```python
from build123d import *

# Parameters (mm, degrees)
SKETCH1_R                = 1.7526
BOSS_EXTRUDE1_DEPTH      = 6.35
BOSS_EXTRUDE2_DEPTH      = 3.175
BOSS_EXTRUDE2_DEPTH_BACK = 3.175


with BuildPart() as part:
    # Sketch1 → Boss-Extrude1 (new body)
    with BuildSketch(Plane.XY):
        with BuildLine():
            Line((-6.345006919, -1.27), (-6.345006919, 37.592))
            ThreePointArc((-6.345006919, 37.592), (0, 43.937006919), (6.345006919, 37.592))
            Line((6.345006919, 37.592), (6.345006919, -1.27))
            ThreePointArc((6.345006919, -1.27), (0, -7.615006919), (-6.345006919, -1.27))
        make_face()
        Circle(SKETCH1_R, mode=Mode.SUBTRACT)
    extrude(amount=BOSS_EXTRUDE1_DEPTH)

    # Sketch2 → Boss-Extrude2 (add, two sides: drawn at the far end of the back side and taken through both)
    with BuildSketch(Plane(origin=(0, 0, 0), x_dir=(0, 0, -1), z_dir=(1, 0, 0)).offset(-BOSS_EXTRUDE2_DEPTH_BACK)):
        with BuildLine():
            Line((0, 37.592), (0, 24.892))
            Line((0, 24.892), (16.951066371, 27.880930353))
            ThreePointArc((16.951066371, 27.880930353), (18.455752886, 28.749661517), (19.05, 30.382342046))
            Line((19.05, 30.382342046), (19.05, 32.101657954))
            ThreePointArc((19.05, 32.101657954), (18.455752886, 33.734338483), (16.951066371, 34.603069647))
            Line((16.951066371, 34.603069647), (0, 37.592))
        make_face()
    extrude(amount=BOSS_EXTRUDE2_DEPTH + BOSS_EXTRUDE2_DEPTH_BACK)


solid = part.part
```
Design review of the part built by this model. Coordinates are the model's own, in mm. A direction names the side the tool comes from. Give positions to 0.01 mm unless a question says otherwise; leave off trailing zeros. Order: outer loops, then holes, each group sorted by start corner. A loop starts at its lowest first (then second) coordinate and runs counter-clockwise, first axis right, second up. Notation, with made-up numbers: (79, 87.25) -> (104, 87.25) arc R13 cw to (104, 106.25) -> close; hole circle Ø6 at (39, 57.25). An arc over 180 degrees is marked (long way). Write item = value, one per line. Start each with the question number.
(1) We need section B-B on x = 0. Write out the cut boundary in (y, z) (3 decimals), plus the area to 3 significant figures.
(2) We need section A-A on y = 0. Write out the cut boundary in (x, z) (3 decimals).
(3) For faces 1 (the face through (-0.044, 36.077, -8.594)), 2 (the face through (3.175, 31, -7)), 3 (the face through (-3.175, 31, -7)), list the 3-axis set-ups (+Z, -Z, +X, -X, +Y, -Y) from which the entire face can be reached by the end or side of a thin tool; tool diameter is ignored.
(4) We need section C-C on z = 1.5. Write out the cut boundary in (x, y) (3 decimals), plus the area to 3 significant figures.
(5) Mouldability with a two-part tool opening along X and no side actions: class faces 4 (the face through (-0.14, 43.935, 3.131)), 5 (the face through (-0.04, 28.73, -18.44)), 6 (the face through (1.67, 0.53, 3.13)) as +X half, -X half, draft (parallel to the pull), parting line (faces both ways), or undercut.
(6) To check wall thickness, follow line 1 along Y through (x, z) = (0, 3) (3 decimals); line 2 along Z through (x, y) = (5.5, 40.5); line 3 along Y through (x, z) = (1, -9.75). State the ranges of each line that lie inside material, in increasing order.
(7) We need section D-D on y = 26. Write out the cut boundary in (x, z) (3 decimals), plus the area to 3 significant figures.
(8) For pin 1 (6 mm diameter, centred on x = -4, z = -2, fed in from +Y); pin 2 (5 mm diameter, centred on x = 4, z = -9.5, fed in from +Y); pin 3 (4 mm diameter, centred on x = -2.5, y = 18.5, fed in from -Z), all flat-tipped, find the tip position at first contact; note any pin that passes through.
Numbers:
q1.outline = (-7.615, 0) -> (-1.753, 0) -> (-1.753, 6.35) -> (-7.615, 6.35) -> close; (1.753, 0) -> (24.892, 0) -> (27.881, -16.951) arc R2.54 ccw to (30.382, -19.05) -> (32.102, -19.05) arc R2.54 ccw to (34.603, -16.951) -> (37.592, 0) -> (43.937, 0) -> (43.937, 6.35) -> (1.753, 6.35) -> close
q1.area = 481 mm^2
q2.outline = (-6.345, 0) -> (-1.753, 0) -> (-1.753, 6.35) -> (-6.345, 6.35) -> close; (1.753, 0) -> (6.345, 0) -> (6.345, 6.35) -> (1.753, 6.35) -> close
q3.face_1 = -Z, +X, -X, +Y
q3.face_2 = -Z, +X, +Y, -Y
q3.face_3 = -Z, -X, +Y, -Y
q4.outline = (-6.345, -1.27) arc R6.345 ccw to (6.345, -1.27) -> (6.345, 37.592) arc R6.345 ccw to (-6.345, 37.592) -> close; hole circle Ø3.505 at (0, 0)
q4.area = 610 mm^2
q5.face_4 = parting line
q5.face_5 = draft
q5.face_6 = undercut
q6.line_1 = -7.615 to -1.753, 1.753 to 43.937
q6.line_2 = 0 to 6.35
q6.line_3 = 26.61 to 35.87
q7.outline = (-6.345, 0) -> (-3.175, 0) -> (-3.175, -6.284) -> (3.175, -6.284) -> (3.175, 0) -> (6.345, 0) -> (6.345, 6.35) -> (-6.345, 6.35) -> close
q7.area = 120 mm^2
q8.pin_1 = 43.69
q8.pin_2 = 36.33
q8.pin_3 = 0
